from build123d import *

# Parameters (mm, degrees)
SKETCH1_W                 = 18.8
SKETCH1_H                 = 34
SKETCH1_R                 = 1.25
CABLE_PLATE_EXTRUDE_DEPTH = 1.4
FILLET2_R                 = 1
FILLET1_R                 = 0.6


with BuildPart() as part:
    # Sketch1 → Cable Plate Extrude (new body)
    with BuildSketch(Plane(origin=(0, 0, 0), x_dir=(1, 0, 0), z_dir=(0, 1, 0))):
        Rectangle(SKETCH1_W, SKETCH1_H)
        with Locations(Location((-7.25, 12.5, 0), (0, 0, 270))):
            Circle(SKETCH1_R, mode=Mode.SUBTRACT)
        with Locations(Location((7.25, 12.5, 0), (0, 0, 270))):
            Circle(SKETCH1_R, mode=Mode.SUBTRACT)
        with Locations(Location((-7.25, -12.5, 0), (0, 0, 270))):
            Circle(SKETCH1_R, mode=Mode.SUBTRACT)
        with Locations(Location((7.25, -12.5, 0), (0, 0, 270))):
            Circle(SKETCH1_R, mode=Mode.SUBTRACT)
    extrude(amount=CABLE_PLATE_EXTRUDE_DEPTH)

    # Fillet2
    fillet2_edges = [part.edges().sort_by_distance(p)[0] for p in [
        (-9.4, 0.7, -17),
        (9.4, 0.7, -17),
        (9.4, 0.7, 17),
        (-9.4, 0.7, 17),
    ]]
    fillet(fillet2_edges, radius=FILLET2_R)

    # Fillet1
    fillet1_edges = [part.edges().sort_by_distance(p)[0] for p in [
        (0, 0, 17),
        (0, 1.4, 17),
        (-9.4, 0, 0),
        (0, 0, -17),
        (9.4, 0, 0),
        (-9.107106781, 0, -16.707106781),
        (9.107106781, 0, -16.707106781),
        (9.107106781, 0, 16.707106781),
        (-9.107106781, 0, 16.707106781),
        (-9.4, 1.4, 0),
        (9.4, 1.4, 0),
        (0, 1.4, -17),
        (-9.107106781, 1.4, -16.707106781),
        (9.107106781, 1.4, -16.707106781),
        (9.107106781, 1.4, 16.707106781),
        (-9.107106781, 1.4, 16.707106781),
    ]]
    fillet(fillet1_edges, radius=FILLET1_R)


solid = part.part
Verification items for the finished model (mm, model axes). Give positions to 0.01 mm unless a question says otherwise; leave off trailing zeros. Loops run counter-clockwise (first coordinate to the right, second up) from the corner with the lowest first, then second, coordinate; pieces in that order, holes last.
1. Cross-section at C-C on y = 1.1. Count the separate pieces of the cut face and the enclosed holes in it, and give its area (3 significant figures).
Derived:
separate pieces: 1
enclosed holes: 4
area: 610 mm2
2. Release check for a two-part mould opening along Z. For faces 1 (the cylindrical face through (-8, 0.7, 11.5)), 2 (the flat face through (0, 0, 0)) record: +Z half, -Z half, draft (parallel to the pull), parting line (faces both ways), or undercut.
Derived:
face 1: undercut
face 2: draft
3. Cross-section at B-B on x = 7.25. Record the cut outline in (y, z).
Derived:
outline: (0, -16.4) arc R0.6 ccw to (0.6, -17) - (0.8, -17) arc R0.6 ccw to (1.4, -16.4) - (1.4, -13.75) - (0, -13.75) - close; (0, -11.25) - (1.4, -11.25) - (1.4, 11.25) - (0, 11.25) - close; (0, 13.75) - (1.4, 13.75) - (1.4, 16.4) arc R0.6 ccw to (0.8, 17) - (0.6, 17) arc R0.6 ccw to (0, 16.4) - close
4. Cross-section at A-A on z = -12.5. Record the cut outline in (x, y), and give its area (3 significant figures).
Derived:
outline: (-9.4, 0.6) arc R0.6 ccw to (-8.8, 0) - (-8.5, 0) - (-8.5, 1.4) - (-8.8, 1.4) arc R0.6 ccw to (-9.4, 0.8) - close; (-6, 0) - (6, 0) - (6, 1.4) - (-6, 1.4) - close; (8.5, 0) - (8.8, 0) arc R0.6 ccw to (9.4, 0.6) - (9.4, 0.8) arc R0.6 ccw to (8.8, 1.4) - (8.5, 1.4) - close
area: 19.0 mm2
5. Material ranges on probe 1 along X at (y, z) = (0.9, -12.5); probe 2 along X at (y, z) = (0.3, -12.5); probe 3 along Z at (x, y) = (5.5, 0.85), recorded low to high.
Derived:
probe 1: x = -9.39 to -8.5, -6 to 6, 8.5 to 9.39
probe 2: x = -9.32 to -8.5, -6 to 6, 8.5 to 9.32
probe 3: z = -17 to 17
